Autodesk Fusion 360 part; units mm, degrees
sketch "Sketch1" plane through (0, 0, 0) normal (1, 0, 0) x (0, 1, 0)
  line L0 (0, 0) -> (10, 0)
  line L1 (10, 0) -> (10, 100)
  line L2 (10, 100) -> (0, 100)
  line L3 (0, 100) -> (0, 0)
  line L4 (5, 0) -> (5, 100) construction
  circle A0 centre (5, 94) radius 3.2
  line L5 (0, 90) -> (10, 90) construction
  circle A1 centre (5, 86) radius 3.2
  arc A2 (0, 0.5051) -> (10, 0.5051) centre (5, 25) ccw
  arc A3 (10, 99.4949) -> (0, 99.4949) centre (5, 75) ccw
  line L6 (0, 50) -> (10, 50) construction
  circle A4 centre (5, 6) radius 3.2
  circle A5 centre (5, 14) radius 3.2
  dimension "d1" = 10
  dimension "d2" = 100
  dimension "d3" = 6.4
  dimension "d4" = 8
  dimension "d11" = 25
  dimension "d20" = 40
extrude "Extrude1" add sketch "Sketch1" along normal blind 4.5 contours L1 L3 A2 A3
extrude "Extrude2" add sketch "Sketch1" along normal up to surface (1.1 mm away) contours A0 | A1 | A4 | A5
sketch "Sketch2" plane through (0, 0, 0) normal (0, 0, 1) x (1, 0, 0)
  line L0 (0, 9.5) -> (4.5, 5.5449)
  line L1 (0, 0) -> (0, 10)
  line L2 (0, 0) -> (0, 10)
  line L3 (0, 0) -> (4.5, 0)
  line L4 (4.5, 0) -> (0, 0)
  line L5 (4.5, 8.2) -> (4.5, 1.8)
  line L6 (4.5, 8.2) -> (4.5, 1.8)
  line L7 (4.5, 8.2) -> (4.5, 1.8)
  line L8 (4.5, 8.2) -> (4.5, 1.8)
  line L9 (4.5, 0) -> (4.5, 10)
  line L10 (4.5, 0) -> (4.5, 10)
  line L11 (0, 10) -> (4.5, 10)
  line L12 (4.5, 10) -> (0, 10)
  line L13 (4.5, 5) -> (0, 5) construction
  line L14 (0, 0.5) -> (4.5, 4.4551)
  dimension "d26" = 0.5
extrude "Extrude3" cut sketch "Sketch2" along normal mid plane 58 from surface at 50 contours L0 L1 L2 L5 L6 L7 L8 L9 L10 L11 L12 | L1 L2 L3 L4 L5 L6 L7 L8 L9 L10 L14
chamfer "Chamfer1" distance 0.5 angle 45 2 edges at (4.5, 2.0166, 95.1572) (4.5, 2.0166, 87.1572)
chamfer "Chamfer3" distance 1 distance2 1 4 edges at (2.25, 0, 99.4949) (2.25, 10, 99.4949) (2.25, 0, 0.5051) (2.25, 10, 0.5051) measured on face at (3, 7.7908, 99.8437) measured on face at (3, 10, 85.8316) measured on face at (3, 0, 14.1684) measured on face at (3, 4.4407, 0.0063)
chamfer "Chamfer2" distance 2 distance2 1 10 edges at (0, 0, 88.7474) (0, 0, 11.2526) (0, 10, 11.2526) (0, 10, 88.7474) (0, 5, 100) (0, 5, 0) (0, 0.4918, 99.0851) (0, 9.5082, 99.0851) (0, 9.5082, 0.9149) (0, 0.4918, 0.9149) measured on face at (1.5, 0, 91.9966) measured on face at (3, 0, 14.5017) measured on face at (3, 10, 8.0034) measured on face at (3, 10, 85.4983) measured on face at (3, 8.1292, 99.8034) measured on face at (3, 4.5518, 0.004) measured on face at (3, 0.6557, 99.2818) measured on face at (3, 9.6721, 98.8884) measured on face at (1.5, 9.6721, 1.1116) measured on face at (1.5, 0.6557, 0.7182)
chamfer "Chamfer4" distance 3.3 angle 45 4 edges at (2.4313, 7.3631, 21) (2.4313, 7.3631, 79) (2.4313, 2.6369, 21) (2.4313, 2.6369, 79)
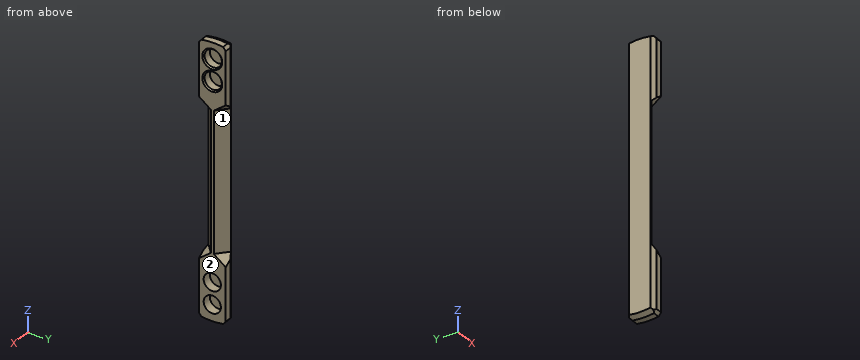
For this review, take the finished solid that the model builds, in its own axes (mm). Face numbers are marked on the shaded views. Round coordinates to 2 decimals unless told otherwise and drop trailing zeros. Loops run counter-clockwise (first coordinate to the right, second up) from the corner with the lowest first, then second, coordinate; pieces in that order, holes last. Notation, with made-up numbers: (70.5, -14) - (75.5, -14) arc R17 cw to (75.5, 4) - close; hole circle Ø8 at (49, 86). An arc over 180 degrees is marked (long way). Put each result on its own line as item: value. Start each with the question number.
1. For probe 1 along Z at (x, y) = (2.55, 5); probe 2 along Z at (x, y) = (4.15, 2.75); probe 3 along Z at (x, y) = (1.15, 7.75), list the stretches that pass through material, from the lowest coordinate up. Write a range as [from, to].
2. Consider section C-C on z = 69. State the section outline as (x, y) points.
3. Insertion check: P1, Ø1.9, axis at y = 5.5, z = 13, coming from the +X side; P2, Ø1, axis at x = 2, y = 7, coming from the -Z side; P3, Ø1.5, axis at x = 0.5, y = 5, coming from the -Z side (3 decimals). Each pin has a flat end and moves straight along its axis. Give the tip position at first contact, or say it passes through.
4. Consider section A-A on z = 6. State the section outline as (x, y) points, plus the area to 3 significant figures.
5. Mouldability with a two-part tool opening along Z and no side actions: class the marked faces 1 and 2 as +Z half, -Z half, draft (parallel to the pull), parting line (faces both ways), or undercut.
6. Consider section B-B on z = 86. State the section outline as (x, y) points, plus the area to 3 significant figures.
Result sheet:
1. probe 1: [0, 2.8], [9.2, 10.8], [17.2, 82.8], [89.2, 90.8], [97.2, 100]
1. probe 2: [0.1, 3.72], [8.28, 11.72], [16.28, 23.25], [76.75, 83.52], [88.48, 91.52], [96.48, 99.9]
1. probe 3: [0.58, 4.36], [7.64, 12.36], [15.64, 84.36], [87.64, 92.36], [95.64, 99.42]
2. outline: (0, 1) - (0.36, 0.82) - (4.5, 4.46) - (4.5, 5.54) - (0.36, 9.18) - (0, 9) - close
3. P1: x = 1.1
3. P2: z = 0.05
3. P3: z = 0.375
4. outline: (0, 1) - (2, 0) - (4.5, 0) - (4.5, 1.8) - (1.1, 1.8) - (1.1, 8.2) - (4.5, 8.2) - (4.5, 10) - (2, 10) - (0, 9) - close
4. area: 21.2 mm^2
5. face 1: undercut
5. face 2: draft
6. outline: (0, 1) - (2, 0) - (4.5, 0) - (4.5, 1.3) - (4, 1.8) - (1.1, 1.8) - (1.1, 8.2) - (4, 8.2) - (4.5, 8.7) - (4.5, 10) - (2, 10) - (0, 9) - close
6. area: 21.0 mm^2
